CAD build for the part. Positions are in the model's coordinates, mm. A direction names the side the tool comes from. Round coordinates to 2 decimals unless told otherwise and drop trailing zeros. Order: outer loops, then holes, each group sorted by start corner. A loop starts at its lowest first (then second) coordinate and runs counter-clockwise, first axis right, second up.
```python
from build123d import *

# Parameters (mm, degrees)
F0_W           = 35
F0_H           = 45
F0_H_2         = 10
F1_DEPTH       = 8
F2_DEPTH       = 5
F3_R           = 4
F4_R           = 3
F5_SIZE        = 10
F7_D           = 5
F7_DEPTH       = 18
F7_CBORE_D     = 10
F7_CBORE_DEPTH = 4
F7_TIP         = 1.5021515476
F8_SIZE        = 1


with BuildPart() as f1:
    # F0 (on Top) → F1 (new body)
    with BuildSketch(Plane.XY):
        Polygon((-17.5, -28.5), (-17.5, 16.5), (-35, 16.5), (-35, -38.5), (-17.5, -38.5), align=None)
        with Locations((0, -6)):
            Rectangle(F0_W, F0_H)
        Polygon((35, 16.5), (17.5, 16.5), (17.5, -28.5), (17.5, -38.5), (35, -38.5), align=None)
        with Locations((0, -33.5)):
            Rectangle(F0_W, F0_H_2)
        with BuildLine():
            Line((9.5, 28.5), (17.5, 28.5))
            ThreePointArc((17.5, 28.5), (0, 46), (-17.5, 28.5))
            Line((-17.5, 28.5), (-9.5, 28.5))
            ThreePointArc((-9.5, 28.5), (0, 38), (9.5, 28.5))
        make_face()
        with BuildLine():
            Line((17.5, 16.5), (17.5, 28.5))
            Line((17.5, 28.5), (9.5, 28.5))
            ThreePointArc((9.5, 28.5), (0, 19), (-9.5, 28.5))
            Line((-9.5, 28.5), (-17.5, 28.5))
            Line((-17.5, 28.5), (-17.5, 16.5))
            Line((-17.5, 16.5), (17.5, 16.5))
        make_face()
    extrude(amount=F1_DEPTH)

    # F0 (on Top) → F2 (join)
    with BuildSketch(Plane.XY):
        with Locations((0, -33.5)):
            Rectangle(F0_W, F0_H_2)
    extrude(amount=-F2_DEPTH)

    # F3
    f3_edges = [f1.edges().sort_by_distance(p)[0] for p in [
        (17.5, -28.5, -2.5),
        (17.5, -38.5, -2.5),
        (-17.5, -28.5, -2.5),
        (-17.5, -38.5, -2.5),
    ]]
    fillet(f3_edges, radius=F3_R)

    # F4
    f4_edges = [f1.edges().sort_by_distance(p)[0] for p in [
        (0, 46, 8),
        (0, 46, 0),
        (9.5, 28.5, 0),
        (9.5, 28.5, 8),
    ]]
    fillet(f4_edges, radius=F4_R)

    # F5
    f5_edges = [f1.edges().sort_by_distance(p)[0] for p in [
        (-35, 16.5, 4),
        (35, 16.5, 4),
        (35, -38.5, 4),
        (-35, -38.5, 4),
    ]]
    chamfer(f5_edges, length=F5_SIZE)

    # F7
    with Locations(Plane.XY.offset(8)):
        with Locations((-27.5, 3), (27.5, 3), (27.5, -22), (-27.5, -22)):
            CounterBoreHole(F7_D / 2, F7_CBORE_D / 2, F7_CBORE_DEPTH, depth=F7_DEPTH)
            with Locations((0, 0, -(F7_DEPTH + F7_TIP / 2))):  # 118° drill point
                Cone(0, F7_D / 2, F7_TIP, mode=Mode.SUBTRACT)

    # F8
    f8_edges = [f1.edges().sort_by_distance(p)[0] for p in [
        (-35, -11, 8),
        (-30, 11.5, 8),
        (-30, -33.5, 8),
        (0, -38.5, 8),
        (30, -33.5, 8),
        (35, -11, 8),
        (30, 11.5, 8),
        (19.75, 16.5, 8),
        (-19.75, 16.5, 8),
    ]]
    chamfer(f8_edges, length=F8_SIZE)


solid = f1.part
```
1. Cut at C-C, the plane x = 27.5. Write the cut outline in (y, z).
2. Cut at A-A, the plane y = 3. Write the cut outline in (x, z), and give its area (3 significant figures).
3. Mould opens along Y. For faces 1 (the face through (-29.71, 11.07, 7.51)), 2 (the face through (16.6, 22.09, 7.14)), 3 (the face through (25, 2, 4)) say: released by +Y, released by -Y, zero draft, split by the parting line, or undercut.
4. Cut at B-B, the plane x = 0. Write the cut outline in (y, z), and give its area (3 significant figures).
5. Tool access for faces 4 (the face through (-30, -23, 4)), 5 (the face through (-16.6, 22.42, 0.86)), 6 (the face through (-17.5, -34, -2)), 7 (the face through (16.297, -37.359, -2.535)): list every direction of +Z, -Z, +X, -X, +Y, -Y with a clear straight run to the whole face (end or side of a thin tool).
6. Drill centre lines: line 1 (Y direction, x = -27.5, z = 6.3); line 2 (X direction, y = 5, z = 6.75); line 3 (X direction, y = 3.5, z = 2). Where is each one in solid material? Low to high.
7. Pin check, flat tips, straight feed: P1, Ø21, axis at x = -13.5, y = 16, coming from the -Z side; P2, Ø1.6, axis at y = 21, z = 4, coming from the +X side; P3, Ø3, axis at x = -27, y = -23, coming from the +Z side. Stop position of each tip, or through.
8. Cut at D-D, the plane z = 1. Write the cut outline in (x, y).
Outcome:
1. outline: (-36, 0) - (-24.5, 0) - (-24.5, 4) - (-27, 4) - (-27, 8) - (-34.59, 8) - (-36, 7) - close; (-19.5, 0) - (0.5, 0) - (0.5, 4) - (-2, 4) - (-2, 8) - (-17, 8) - (-17, 4) - (-19.5, 4) - close; (5.5, 0) - (14, 0) - (14, 7) - (12.59, 8) - (8, 8) - (8, 4) - (5.5, 4) - close
2. outline: (-35, 0) - (-30, 0) - (-30, 4) - (-32.5, 4) - (-32.5, 8) - (-34, 8) - (-35, 7) - close; (-25, 0) - (25, 0) - (25, 4) - (22.5, 4) - (22.5, 8) - (-22.5, 8) - (-22.5, 4) - (-25, 4) - close; (30, 0) - (35, 0) - (35, 7) - (34, 8) - (32.5, 8) - (32.5, 4) - (30, 4) - close
2. area: 439 mm2
3. face 1: released by +Y
3. face 2: zero draft
3. face 3: undercut
4. outline: (-38.5, -5) - (-28.5, -5) - (-28.5, 0) - (16, 0) arc R3 ccw to (19, 3) - (19, 5) arc R3 ccw to (16, 8) - (-37.5, 8) - (-38.5, 7) - close; (38, 3) arc R3 ccw to (41, 0) - (43, 0) arc R3 ccw to (46, 3) - (46, 5) arc R3 ccw to (43, 8) - (41, 8) arc R3 ccw to (38, 5) - close
4. area: 562 mm2
5. face 4: +Z
5. face 5: -Z, -X, +Y
5. face 6: -Z, -X, +Y, -Y
5. face 7: -Z, +X, -Y
6. line 1: y = -36 to -27, -17 to -2, 8 to 14
6. line 2: x = -35 to -32.08, -22.92 to 22.92, 32.08 to 35
6. line 3: x = -35 to -29.95, -25.05 to 25.05, 29.95 to 35
7. P1: stops at z = 0
7. P2: stops at x = 17.5
7. P3: stops at z = 4
8. outline: (-35, -28.5) - (-25, -38.5) - (25, -38.5) - (35, -28.5) - (35, 6.5) - (25, 16.5) - (16.74, 16.5) - (16.74, 28.5) arc R16.74 ccw to (-16.74, 28.5) - (-16.74, 16.5) - (-25, 16.5) - (-35, 6.5) - close; hole circle Ø5 at (-27.5, -22); hole circle Ø5 at (-27.5, 3); hole circle Ø20.53 at (0, 28.5); hole circle Ø5 at (27.5, -22); hole circle Ø5 at (27.5, 3)
